from build123d import *

# Parameters (mm, degrees)
SKETCH1_R                  = 8.5
BOSS_EXTRUDE1_DEPTH        = 5.5
BOSS_EXTRUDE2_DEPTH        = 4
BOSS_EXTRUDE2_DEPTH_BACK   = 0.4
SKETCH2_R                  = 10
SKETCH3_R                  = 3
CUT_EXTRUDE1_DEPTH         = 18.426201537
SKETCH6_R                  = 1
CUT_EXTRUDE4_DEPTH         = 18.426201537
F_3_2_3_2_DIAMETER_HOLE1_D = 3.2
SKETCH10_R                 = 1.95
CUT_EXTRUDE5_DEPTH         = 4
CHAMFER1_SIZE              = 0.3


with BuildPart() as part:
    # Sketch1 → Boss-Extrude1 (new body)
    with BuildSketch(Plane(origin=(0, 0, 0), x_dir=(1, 0, 0), z_dir=(0, 1, 0))):
        with Locations(Location((0, 0, 0), (0, 0, 270))):
            Circle(SKETCH1_R)
    extrude(amount=BOSS_EXTRUDE1_DEPTH)

    # Sketch2 → Boss-Extrude2 (add, two sides: drawn at the far end of the back side and taken through both)
    with BuildSketch(Plane(origin=(0, 5.5, 0), x_dir=(1, 0, 0), z_dir=(0, 1, 0)).offset(-BOSS_EXTRUDE2_DEPTH_BACK)):
        with Locations(Location((-0.65, 0, 0), (0, 0, 270))):
            Circle(SKETCH2_R)
    extrude(amount=BOSS_EXTRUDE2_DEPTH + BOSS_EXTRUDE2_DEPTH_BACK)

    # Sketch3 → Cut-Extrude1 (cut, through all)
    with BuildSketch(Plane.XZ):
        with Locations(Location((-0.65, 0, 0), (0, 0, 270))):
            Circle(SKETCH3_R)
    extrude(amount=-CUT_EXTRUDE1_DEPTH, mode=Mode.SUBTRACT)

    # Sketch6 → Cut-Extrude4 (cut, through all)
    with BuildSketch(Plane.XZ):
        with Locations(Location((4.35, 0, 0), (0, 0, 270))):
            Circle(SKETCH6_R)
    extrude(amount=-CUT_EXTRUDE4_DEPTH, mode=Mode.SUBTRACT)

    # Ø3.2 (3.2) Diameter Hole1 (through all)
    with Locations(Plane(origin=(0, 0, 0), x_dir=(-1, 0, 0), z_dir=(0, -1, 0))):
        with Locations((0.65, 6.5), (0.65, -6.5)):
            Hole(F_3_2_3_2_DIAMETER_HOLE1_D / 2)

    # Sketch10 → Cut-Extrude5 (cut)
    with BuildSketch(Plane(origin=(0, 9.5, 0), x_dir=(1, 0, 0), z_dir=(0, 1, 0))):
        with Locations(Location((-0.65, 6.5, 0), (0, 0, 270))):
            Circle(SKETCH10_R)
        with Locations(Location((-0.65, -6.5, 0), (0, 0, 270))):
            Circle(SKETCH10_R)
    extrude(amount=-CUT_EXTRUDE5_DEPTH, mode=Mode.SUBTRACT)

    # Chamfer1
    chamfer1_edges = [part.edges().sort_by_distance(p)[0] for p in [
        (-0.65, 9.5, 3),
        (-0.65, 0, 3),
        (4.35, 9.5, 1),
        (4.35, 0, 1),
        (-2.25, 0, 6.5),
        (-2.25, 0, -6.5),
        (-0.65, 9.5, -8.45),
        (-0.65, 9.5, 4.55),
    ]]
    chamfer(chamfer1_edges, length=CHAMFER1_SIZE)


solid = part.part
Check sheet for the modelled part. Datum: model origin and axes. Units: mm. A direction names the side the tool comes from. Give positions to 0.01 mm unless a question says otherwise; leave off trailing zeros. Loops run counter-clockwise (first coordinate to the right, second up) from the corner with the lowest first, then second, coordinate; pieces in that order, holes last. Notation, with made-up numbers: M 36,82.25 L 75,82.25 A27 ccw 75,110.25 Z; hole C -0.75,-2 d9. An arc over 180 degrees is marked long. Answer as a JSON object with one key per item and string values. Group by question number.
Q1. Material ranges on line 1 along Z through (x, y) = (-1.5, 3); line 2 along Z through (x, y) = (-0.5, 1.25); line 3 along Y through (x, z) = (-9.5, 2), recorded low to high. Write a range as [from, to].
Q2. Go/stop test with flat-tipped pins: P1, Ø3, axis at x = -1.5, z = 6, coming from the +Y side; P2, Ø4, axis at y = 2, z = -5.5, coming from the -X side; P3, Ø2, axis at y = 1, z = 0.5, coming from the +X side; P4, Ø3, axis at y = 2.5, z = 0, coming from the -X side. Record where each tip stops, or that it passes through.
Q3. Cross-section at D-D on z = -6.5. Record the cut outline in (x, y).
Q4. Cross-section at A-A on y = 1. Record the cut outline in (x, z).
Q5. Cross-section at B-B on z = 0. Record the cut outline in (x, y), then the cut area to 3 significant figures.
Q6. Cross-section at C-C on x = 4.35. Record the cut outline in (y, z).
Q7. Release check for a two-part mould opening along Z. For faces 1 (the flat face through (0, 0, 4)), 2 (the cylindrical face through (-1.8, 4.69, -2.77)), 3 (the cylindrical face through (8.428, 2.514, -1.107)) record: released by +Z, released by -Z, zero draft, split by the parting line, or undercut.
Q8. Access from +Z, -Z, +X, -X, +Y, -Y to the whole of each face (thin tool, end or side, straight path). Record for faces 4 (the cylindrical face through (-0.564, 7.376, 4.552)), 5 (the flat face through (-9, 5.1, 0)), 6 (the flat face through (-5, 9.5, 0)).
Evaluation:
{
 "1": {"line 1": "z = [-8.37, -7.86], [-5.14, -2.88], [2.88, 5.14], [7.86, 8.37]", "line 2": "z = [-8.49, -8.09], [-4.91, -3], [3, 4.91], [8.09, 8.49]", "line 3": "y = [5.1, 9.5]"},
 "2": {"P1": "stops at y = 9.5", "P2": "stops at x = -7.75", "P3": "stops at x = 8.5", "P4": "stops at x = -8.5"},
 "3": {"outline": "M -8.25,5.1 L -5.48,5.1 L -5.48,0 L -2.55,0 L -2.25,0.3 L -2.25,5.5 L -2.6,5.5 L -2.6,9.2 L -2.9,9.5 L -8.25,9.5 Z; M 0.95,0.3 L 1.25,0 L 5.48,0 L 5.48,5.1 L 6.95,5.1 L 6.95,9.5 L 1.6,9.5 L 1.3,9.2 L 1.3,5.5 L 0.95,5.5 Z"},
 "4": {"outline": "C 0,0 d17; hole C -0.65,0 d6; hole C -0.65,-6.5 d3.2; hole C -0.65,6.5 d3.2; hole C 4.35,0 d2"},
 "5": {"outline": "M -10.65,5.1 L -8.5,5.1 L -8.5,0 L -3.95,0 L -3.65,0.3 L -3.65,9.2 L -3.95,9.5 L -10.65,9.5 Z; M 2.35,0.3 L 2.65,0 L 3.05,0 L 3.35,0.3 L 3.35,9.2 L 3.05,9.5 L 2.65,9.5 L 2.35,9.2 Z; M 5.35,0.3 L 5.65,0 L 8.5,0 L 8.5,5.1 L 9.35,5.1 L 9.35,9.5 L 5.65,9.5 L 5.35,9.2 Z", "area": "98.3 mm2"},
 "6": {"outline": "M 0,-7.3 L 5.1,-7.3 L 5.1,-8.66 L 9.5,-8.66 L 9.5,-1.3 L 9.2,-1 L 0.3,-1 L 0,-1.3 Z; M 0,1.3 L 0.3,1 L 9.2,1 L 9.5,1.3 L 9.5,8.66 L 5.1,8.66 L 5.1,7.3 L 0,7.3 Z"},
 "7": {"face 1": "zero draft", "face 2": "undercut", "face 3": "split by the parting line"},
 "8": {"face 4": "+Y", "face 5": "-Y", "face 6": "+Z, -Z, +X, -X, +Y"}
}
